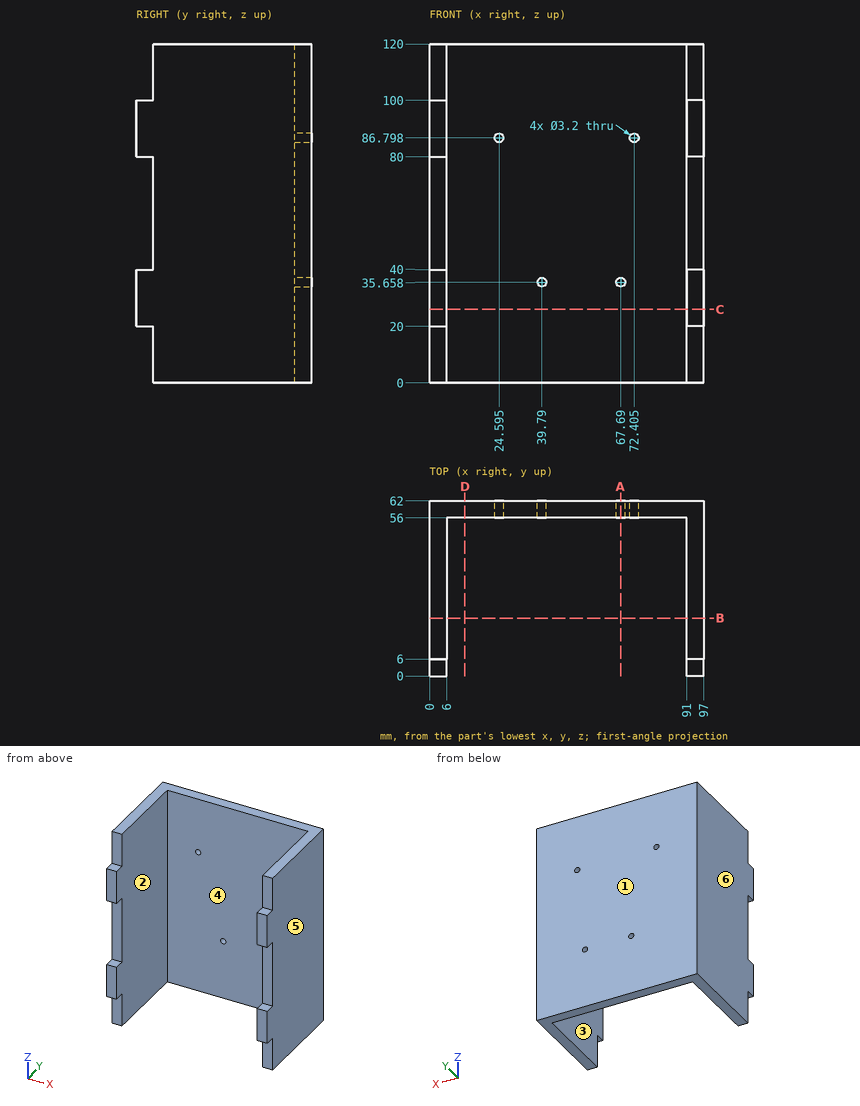
Geometry: see drawing. Coordinates: mm, zero at the bounding-box minimum. A direction names the side the tool comes from. Coordinates: 2 decimals unless noted, no trailing zeros. Loops run counter-clockwise (first coordinate to the right, second up) from the corner with the lowest first, then second, coordinate; pieces in that order, holes last. Notation, with made-up numbers: (30.5, 43.25) - (79.5, 43.25) arc R18 ccw to (79.5, 58.25) - close; hole circle Ø5 at (33.5, 19.5). An arc over 180 degrees is marked (long way). Answer as CSV lines item,"result".
1. Section D-D (x = 12.5). Return loops of the section in (y, z).
Established:
outline,"(56, 0) - (62, 0) - (62, 120) - (56, 120) - close"
2. Contact query for flat-ended pins moving along their axis: pin 1 (1.8 mm diameter, centred on x = 2.5, z = 114, fed in from -Y); pin 2 (1.8 mm diameter, centred on x = 93, y = 3.5, fed in from -Z); pin 3 (5 mm diameter, centred on x = 16, z = 50.5, fed in from -Y). Output: stop coordinate, or through.
Established:
pin 1,"stops at y = 6"
pin 2,"stops at z = 20"
pin 3,"stops at y = 56"
3. Mould query, pull axis X, two halves, no side actions, for the marked faces 3, 4, 5 and 6. Classes: released by +X, released by -X, zero draft, split by the parting line, or undercut.
Established:
face 3,"undercut"
face 4,"undercut"
face 5,"released by +X"
face 6,"released by -X"
4. Section A-A (x = 67.69). Return loops of the section in (y, z), then the cut area to 3 significant figures.
Established:
outline,"(56, 0) - (62, 0) - (62, 34.06) - (56, 34.06) - close; (56, 37.26) - (62, 37.26) - (62, 120) - (56, 120) - close"
area,"701 mm2"
5. Section B-B (y = 20.5). Return loops of the section in (x, z), then the cut area to 3 significant figures.
Established:
outline,"(0, 0) - (6, 0) - (6, 120) - (0, 120) - close; (91, 0) - (97, 0) - (97, 120) - (91, 120) - close"
area,"1,440 mm2"
6. Section C-C (z = 26). Return loops of the section in (x, y).
Established:
outline,"(0, 0) - (6, 0) - (6, 56) - (91, 56) - (91, 0) - (97, 0) - (97, 62) - (0, 62) - close"
7. Reachability of the marked faces 1 and 2 from +Z, -Z, +X, -X, +Y, -Y: full face, straight path, thin tool, end or side. Return the list, or none.
Established:
face 1,"+Z, -Z, +X, -X, +Y"
face 2,"+Z, -Z, -Y"
8. Ray query, line 1 (X direction, y = 36.5, z = 83.5); line 2 (Y direction, x = 29, z = 113). Return the intervals inside material, ascending.
Established:
line 1,"x = 0 to 6, 91 to 97"
line 2,"y = 56 to 62"
